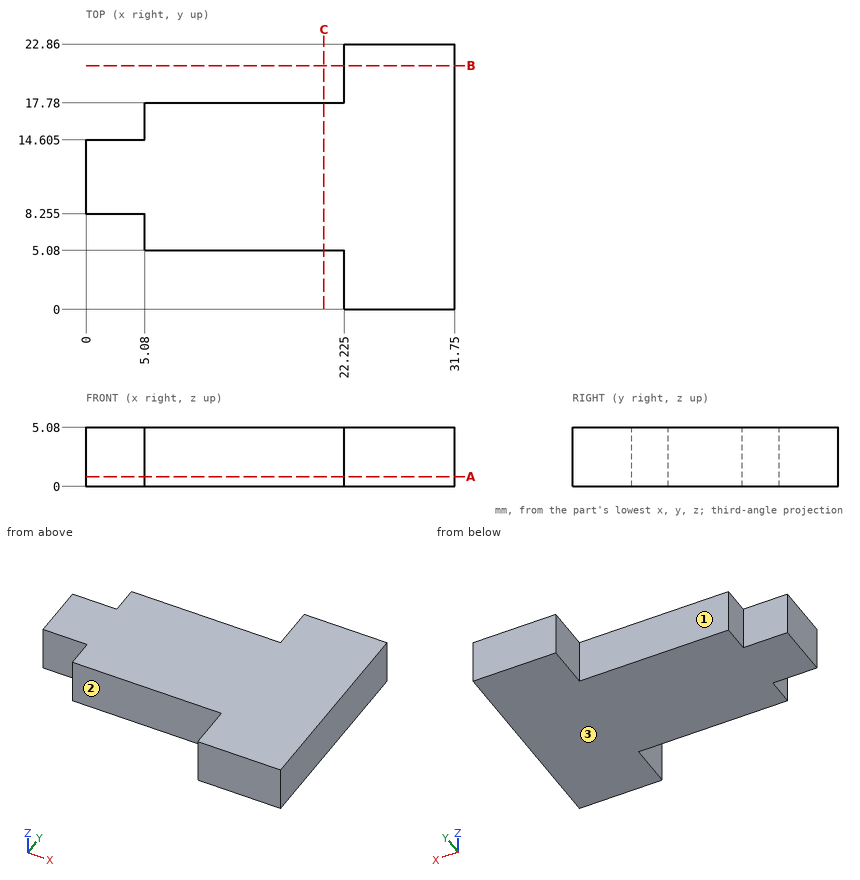
Here's the drawing with two shaded views (mm, measured from the low corner). I have some questions. A direction names the side the tool comes from. Coordinates: 2 decimals unless noted, no trailing zeros. Order: outer loops, then holes, each group sorted by start corner. A loop starts at its lowest first (then second) coordinate and runs counter-clockwise, first axis right, second up. Notation, with made-up numbers: (76.5, 56) - (111.5, 56) arc R30 ccw to (111.5, 81) - close; hole circle Ø11 at (-5.5, 15). An arc over 180 degrees is marked (long way). Use CSV: the item, a comma, the result in double quotes. Start each with the question number.
1. I'm going to push flat-ended pins straight in: pin 1 (2.5 mm diameter, centred on y = 2.5, z = 3.5, fed in from -X) (3 decimals); pin 2 (2.5 mm diameter, centred on x = 3, z = 3.5, fed in from -Y) (3 decimals); pin 3 (12 mm diameter, centred on x = 11.5, y = 7, fed in from -Z); pin 4 (1.5 mm diameter, centred on x = 19, z = 4, fed in from -Y). Where does each tip first touch, or does it pass through?
2. Suppose I cut it at A-A on z = 0.85. List the corners of the cut face in (x, y) for me (3 decimals), then the cut area to 3 significant figures.
3. Suppose I cut it at B-B on y = 21. List the corners of the cut face in (x, z) for me (3 decimals), then the cut area to 3 significant figures.
4. For the marked faces 1, 2 and 3, which set-ups out of +Z, -Z, +X, -X, +Y, -Y let a thin tool reach every point of the face, with its end or its side?
5. Please list where these lines run through material, in increasing order: line 1 (X direction, y = 1.25, z = 3.4) (3 decimals); line 2 (Y direction, x = 3, z = 1.6) (3 decimals); line 3 (Y direction, x = 11, z = 1.1). Write a range as from..to.
6. Suppose I cut it at C-C on x = 20.5. List the corners of the cut face in (y, z) for me.
Output:
1,pin 1,"stops at x = 22.225"
1,pin 2,"stops at y = 8.255"
1,pin 3,"stops at z = 0"
1,pin 4,"stops at y = 5.08"
2,outline,"(0, 8.255) - (5.08, 8.255) - (5.08, 5.08) - (22.225, 5.08) - (22.225, 0) - (31.75, 0) - (31.75, 22.86) - (22.225, 22.86) - (22.225, 17.78) - (5.08, 17.78) - (5.08, 14.605) - (0, 14.605) - close"
2,area,"468 mm2"
3,outline,"(22.225, 0) - (31.75, 0) - (31.75, 5.08) - (22.225, 5.08) - close"
3,area,"48.4 mm2"
4,face 1,"+Z, -Z, -X, +Y"
4,face 2,"+Z, -Z, -X, -Y"
4,face 3,"-Z, +X, -X, +Y, -Y"
5,line 1,"x = 22.225..31.75"
5,line 2,"y = 8.255..14.605"
5,line 3,"y = 5.08..17.78"
6,outline,"(5.08, 0) - (17.78, 0) - (17.78, 5.08) - (5.08, 5.08) - close"
